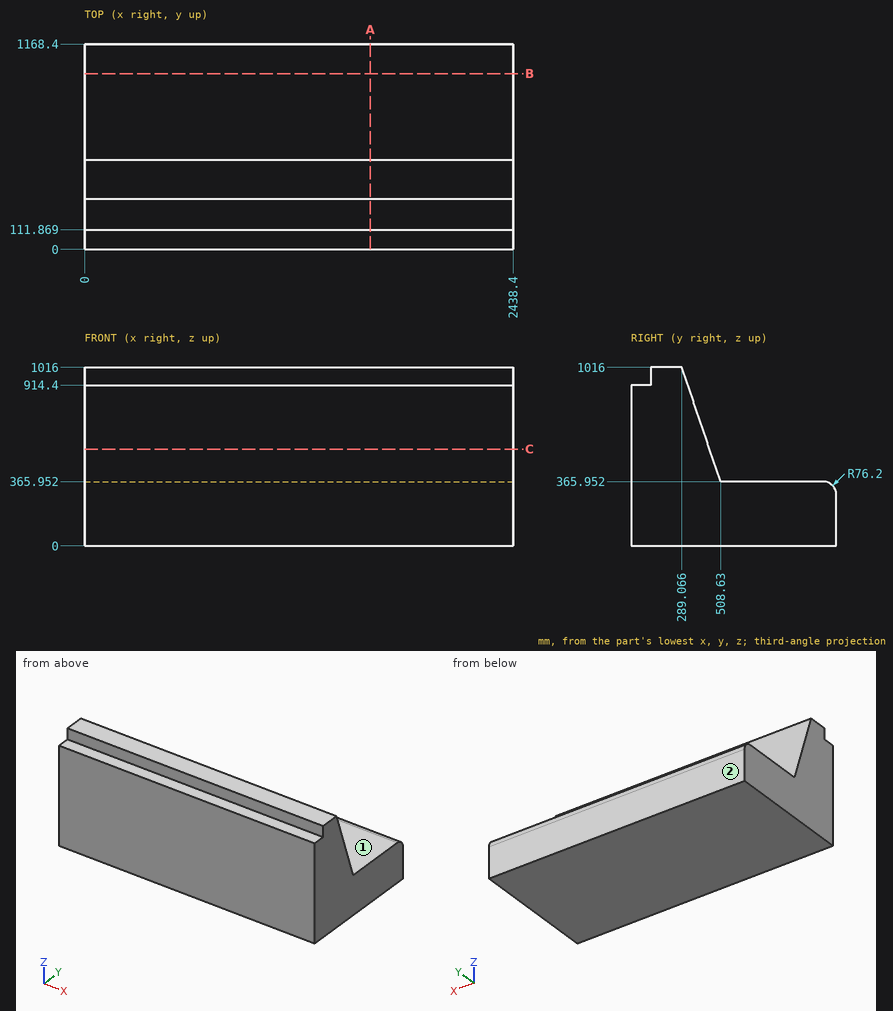
Geometry check sheet. Reference: drawing and pictorial views, mm from the part's lowest x, y, z. A direction names the side the tool comes from. Coordinates: 2 decimals unless noted, no trailing zeros. Order: outer loops, then holes, each group sorted by start corner. A loop starts at its lowest first (then second) coordinate and runs counter-clockwise, first axis right, second up. Notation, with made-up numbers: (24, -40) - (54, -40) arc R28 ccw to (54, -21) - close; hole circle Ø3 at (79.25, 20). An arc over 180 degrees is marked (long way). Answer in a Markdown table with one row per item. Add a question column.
1) Cross-section at B-B, the plane y = 1000. Record the cut outline in (x, z), then the cut area to 3 significant figures.
2) Gauge pin test, flat ends, axial feed: P1, Ø5, axis at x = 2084, y = 1027, coming from the +Z side; P2, Ø8, axis at x = 1274.5, z = 592.5, coming from the -Y side; P3, Ø12, axis at x = 732.5, z = 813, coming from the +Y side; P4, Ø12, axis at x = 1289.5, z = 686.5, coming from the +Y side (1 decimal). Record the tip position at first contact, or that the pin passes through.
3) Cross-section at C-C, the plane z = 550.5. Record the cut outline in (x, y) (1 decimal), then the cut area to 3 significant figures.
4) Set-up check for the marked faces 1 and 2: record each of +Z, -Z, +X, -X, +Y, -Y from which the full face is reachable in a straight line by a thin tool's end or side.
5) Material ranges on line 1 along Z through (x, y) = (897, 789); line 2 along Z through (x, y) = (167.5, 51); line 3 along Y through (x, z) = (2335.5, 475), recorded low to high. Write a range as [from, to].
6) Cross-section at A-A, the plane x = 1627. Record the cut outline in (y, z) (1 decimal), then the cut area to 3 significant figures.
Check result:
| question | item | result |
|---|---|---|
| 1 | outline | (0, 0) - (2438.4, 0) - (2438.4, 365.95) - (0, 365.95) - close |
| 1 | area | 892,000 mm² |
| 2 | P1 | stops at z = 365.95 |
| 2 | P2 | stops at y = 0 |
| 2 | P3 | stops at y = 359.66 |
| 2 | P4 | stops at y = 402.4 |
| 3 | outline | (0, 0) - (2438.4, 0) - (2438.4, 446.3) - (0, 446.3) - close |
| 3 | area | 1,090,000 mm² |
| 4 | face 1 | +Z, +X, -X, +Y |
| 4 | face 2 | +Z, -Z, +X, -X, +Y |
| 5 | line 1 | z = [0, 365.95] |
| 5 | line 2 | z = [0, 914.4] |
| 5 | line 3 | y = [0, 471.8] |
| 6 | outline | (0, 0) - (1168.4, 0) - (1168.4, 289.8) arc R76.2 ccw to (1092.2, 366) - (508.6, 366) - (289.1, 1016) - (111.9, 1016) - (111.9, 914.4) - (0, 914.4) - close |
| 6 | area | 674,000 mm² |
